from build123d import *

# Parameters (mm, degrees)
F1_DEPTH = 7


with BuildPart() as f1:
    # F0 (on Top) → F1 (new body)
    with BuildSketch(Plane.XY):
        with BuildLine():
            Line((-7, -3), (0, -3))
            ThreePointArc((0, -3), (-1.5, -2.5980762114), (-2.5980762114, -1.5))
            Line((-2.5980762114, -1.5), (-7, -1.5))
            Line((-7, -1.5), (-7, -3))
        make_face()
        with BuildLine():
            Line((-2.5980762114, -1.5), (0, -1.5))
            Line((0, -1.5), (0, -3))
            ThreePointArc((0, -3), (2.1213203436, -2.1213203436), (3, 0))
            ThreePointArc((3, 0), (-0.7764571353, 2.8977774789), (-2.5980762114, -1.5))
        make_face()
        with BuildLine():
            ThreePointArc((0, -1.5), (-1.0606601718, 1.0606601718), (1.5, 0))
            ThreePointArc((1.5, 0), (1.0606601718, -1.0606601718), (0, -1.5))
        make_face(mode=Mode.SUBTRACT)
        with BuildLine():
            Line((0, -3), (0, -1.5))
            Line((0, -1.5), (-2.5980762114, -1.5))
            ThreePointArc((-2.5980762114, -1.5), (-1.5, -2.5980762114), (0, -3))
        make_face()
    extrude(amount=F1_DEPTH)


solid = f1.part
Geometry check sheet. Reference: the model listing, model coordinates, mm. Coordinates: 2 decimals unless noted, no trailing zeros. Loops run counter-clockwise (first coordinate to the right, second up) from the corner with the lowest first, then second, coordinate; pieces in that order, holes last. Notation, with made-up numbers: (-36, 60) - (3, 60) arc R19 cw to (3, 78) - close; hole circle Ø10 at (-38, -24). An arc over 180 degrees is marked (long way). Use one line per item in the form item = value. Start each with the question number.
Item 1: Section check C-C, the plane y = -0.5. Enter the section's corners in (x, z), and give its area (3 significant figures).
Item 2: Section check B-B, the plane z = 5.25. Enter the section's corners in (x, y).
Item 3: Section check A-A, the plane x = -0.25. Enter the section's corners in (y, z), and give its area (3 significant figures).
Item 4: Gauge pin test, flat ends, axial feed: pin 1 (3 mm diameter, centred on x = -4.5, y = -1, fed in from -Z); pin 2 (2.5 mm diameter, centred on x = 0, y = 0, fed in from -Z) (3 decimals); pin 3 (3 mm diameter, centred on x = 2, z = 2.5, fed in from +Y); pin 4 (2 mm diameter, centred on x = -4.5, z = 2, fed in from +Y). Record the tip position at first contact, or that the pin passes through.
Item 5: Thickness scan on probe 1 along X at (y, z) = (0, 4); probe 2 along X at (y, z) = (1, 2.25); probe 3 along Y at (x, z) = (0.25, 2.5). Record the ranges inside material, lowest first.
Item 6: Section check D-D, the plane x = -4.25. Enter the section's corners in (y, z), and give its area (3 significant figures).
Computed:
q1.outline = (-2.96, 0) - (-1.41, 0) - (-1.41, 7) - (-2.96, 7) - close; (1.41, 0) - (2.96, 0) - (2.96, 7) - (1.41, 7) - close
q1.area = 21.6 mm2
q2.outline = (-7, -3) - (0, -3) arc R3 ccw (long way) to (-2.6, -1.5) - (-7, -1.5) - close; hole circle Ø3 at (0, 0)
q3.outline = (-3, 0) - (-1.48, 0) - (-1.48, 7) - (-3, 7) - close; (1.48, 0) - (2.99, 0) - (2.99, 7) - (1.48, 7) - close
q3.area = 21.2 mm2
q4.pin_1 = 0
q4.pin_2 = through
q4.pin_3 = 2.96
q4.pin_4 = -1.5
q5.probe_1 = -3 to -1.5, 1.5 to 3
q5.probe_2 = -2.83 to -1.12, 1.12 to 2.83
q5.probe_3 = -2.99 to -1.48, 1.48 to 2.99
q6.outline = (-3, 0) - (-1.5, 0) - (-1.5, 7) - (-3, 7) - close
q6.area = 10.5 mm2
